Can you work these out from the model? Positions are in its coordinate system, mm. Face numbers are marked on the shaded views. A direction names the side the tool comes from. Give positions to 0.01 mm unless a question says otherwise; leave off trailing zeros. Order: outer loops, then holes, each group sorted by start corner. A loop starts at its lowest first (then second) coordinate and runs counter-clockwise, first axis right, second up. Notation, with made-up numbers: (-38, 79.25) - (13, 79.25) arc R28 ccw to (13, 115.25) - close; hole circle Ø11 at (38, -35). An arc over 180 degrees is marked (long way). Use one line per item in the form item = value. Start each with the question number.
1) Suppose I cut it at D-D, the plane x = 8.5. Write out the boundary of the cut face in (y, z).
2) Suppose I cut it at C-C, the plane y = 2.25. Write out the boundary of the cut face in (x, z), and give its area (3 significant figures).
3) Suppose I cut it at A-A, the plane z = 63.5. Write out the boundary of the cut face in (x, y) (1 decimal), and give its area (3 significant figures).
4) Please list where these lines run through material, in increasing order: probe 1 along X at (y, z) = (4, 28); probe 2 along Z at (x, y) = (41, 3); probe 3 along Z at (x, y) = (70, 1.25).
5) Which directions (+Z, -Z, +X, -X, +Y, -Y) give clear straight access to the entire face, cutting with the end or side of a thin tool? Please do the marked faces 1, 2 and 3.
6) For pin 1 (6 mm diameter, centred on x = 32.5, y = 7.5, fed in from +Z); pin 2 (10 mm diameter, centred on x = 44, z = 8.5, fed in from +Y) (3 decimals); pin 3 (8 mm diameter, centred on x = 11, y = 8, fed in from +Z); pin 4 (4 mm diameter, centred on y = 12.5, z = 38.5, fed in from +X), each with a flat end and sliding along its axis, tell me the tip position at first contact or that it passes through.
7) We'd pull the mould along Z, two halves only. Please class the marked faces 4, 5, 6 and 7: released by +Z, released by -Z, zero draft, split by the parting line, or undercut.
8) Suppose I cut it at B-B, the plane x = 54.5. Write out the boundary of the cut face in (y, z), and give its area (3 significant figures).
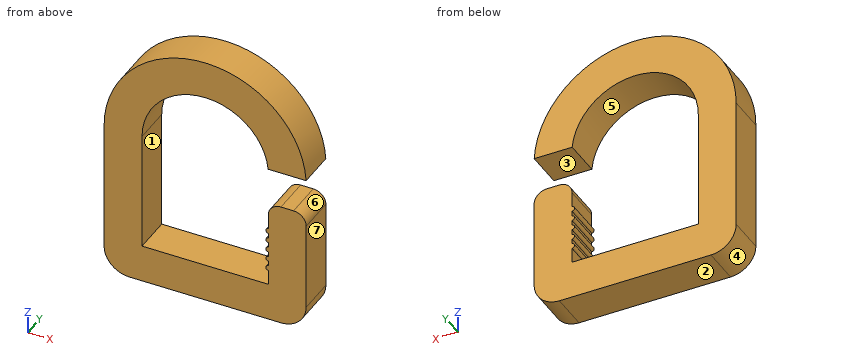
```python
from build123d import *

# Parameters (mm, degrees)
BOSS_EXTRUDE1_DEPTH = 15
FILLET2_R           = 10
FILLET3_R           = 5
SKETCH3_R           = 1
BOSS_EXTRUDE2_DEPTH = 15


with BuildPart() as part:
    # Sketch2 → Boss-Extrude1 (new body)
    with BuildSketch(Plane(origin=(0, 0, 0), x_dir=(1, 0, 0), z_dir=(0, 1, 0))):
        with BuildLine():
            Line((64.937954364, -49.659577053), (79.978719708, -49.659577053))
            ThreePointArc((79.978719708, -49.659577053), (38.858723791, -87.337822877), (0, -47.331525149))
            Line((0, -47.331525149), (0, 0))
            Line((0, 0), (0, 15))
            Line((0, 15), (80, 15))
            Line((80, 15), (80, 0))
            Line((80, 0), (80, -35))
            Line((80, -35), (65, -35))
            Line((65, -35), (65, 0))
            Line((65, 0), (15, 0))
            Line((15, 0), (15, -47.331525149))
            ThreePointArc((15, -47.331525149), (38.857952611, -72.327620402), (64.937954364, -49.659577053))
        make_face()
    extrude(amount=BOSS_EXTRUDE1_DEPTH)

    # Fillet2
    fillet2_edges = [part.edges().sort_by_distance(p)[0] for p in [
        (0, 7.5, -15),
        (80, 7.5, -15),
    ]]
    fillet(fillet2_edges, radius=FILLET2_R)

    # Fillet3
    fillet3_edges = [part.edges().sort_by_distance(p)[0] for p in [
        (80, 7.5, 35),
        (65, 7.5, 35),
    ]]
    fillet(fillet3_edges, radius=FILLET3_R)

    # Sketch3 → Boss-Extrude2 (add)
    with BuildSketch(Plane(origin=(0, 15, 0), x_dir=(1, 0, 0), z_dir=(0, 1, 0))):
        with Locations((65, -15)):
            Circle(SKETCH3_R)
        with Locations((65, -11)):
            Circle(SKETCH3_R)
        with Locations((65, -23)):
            Circle(SKETCH3_R)
        with Locations((65, -19)):
            Circle(SKETCH3_R)
        with Locations((65, -7)):
            Circle(SKETCH3_R)
    extrude(amount=-BOSS_EXTRUDE2_DEPTH)


solid = part.part
```
Result sheet:
q1.outline = (0, -14.89) - (15, -14.89) - (15, 71.99) - (0, 71.99) - close
q2.outline = (0, -5) arc R10 ccw to (10, -15) - (70, -15) arc R10 ccw to (80, -5) - (80, 30) arc R5 ccw to (75, 35) - (70, 35) arc R5 ccw to (65, 30) - (65, 24) arc R1 ccw to (65, 22) - (65, 20) arc R1 ccw to (65, 18) - (65, 16) arc R1 ccw to (65, 14) - (65, 12) arc R1 ccw to (65, 10) - (65, 8) arc R1 ccw to (65, 6) - (65, 0) - (15, 0) - (15, 47.33) arc R25.02 cw to (64.94, 49.66) - (79.98, 49.66) arc R40.02 ccw to (0, 47.33) - close
q2.area = 3,890 mm²
q3.outline = (3.4, 0) - (20.9, 0) - (20.9, 15) - (3.4, 15) - close; (59.1, 0) - (76.6, 0) - (76.6, 15) - (59.1, 15) - close
q3.area = 525 mm²
q4.probe_1 = 0 to 15, 65 to 80
q4.probe_2 = -15 to 0, 72.34 to 87.34
q4.probe_3 = -15 to 35, 49.66 to 73.85
q5.face_1 = +Y, -Y
q5.face_2 = -Z, +X, -X, +Y, -Y
q5.face_3 = +X, +Y, -Y
q6.pin_1 = 87.1
q6.pin_2 = through
q6.pin_3 = 78.57
q6.pin_4 = 15
q7.face_4 = released by -Z
q7.face_5 = undercut
q7.face_6 = undercut
q7.face_7 = zero draft
q8.outline = (0, -15) - (15, -15) - (15, 0) - (0, 0) - close; (0, 67.74) - (15, 67.74) - (15, 84.64) - (0, 84.64) - close
q8.area = 479 mm²
